```python
from build123d import *

# Parameters (mm, degrees)
F0_R     = 12
F0_R_2   = 10.25
F1_DEPTH = 270
F2_R     = 12
F3_DEPTH = 5
F4_R     = 12
F5_DEPTH = 5


with BuildPart() as f1:
    # F0 (on Front) → F1 (new body)
    with BuildSketch(Plane.XZ):
        Circle(F0_R)
        Circle(F0_R_2, mode=Mode.SUBTRACT)
    extrude(amount=F1_DEPTH)

    # F2 (on face) → F3 (join)
    with BuildSketch(Plane(origin=(0, 0, 0), x_dir=(-1, 0, 0), z_dir=(0, 1, 0))):
        Circle(F2_R)
    extrude(amount=F3_DEPTH)

    # F4 (on face) → F5 (join)
    with BuildSketch(Plane.XZ.offset(270)):
        Circle(F4_R)
    extrude(amount=F5_DEPTH)


solid = f1.part
```
Work out the finished part from the listing and answer in its coordinate system (mm). Round coordinates to 2 decimals unless told otherwise and drop trailing zeros. Write each loop counter-clockwise with the first axis right and the second up, starting at its lowest first coordinate (ties: lowest second). Pieces come first, ordered by that corner, then holes. Notation, with made-up numbers: (37, -3.5) -> (63, -3.5) arc R8 ccw to (63, 9.5) -> close; hole circle Ø8 at (-32, -40). An arc over 180 degrees is marked (long way). Write each question's results on one line, items separated by ' | '.
1) Flat-ended cylindrical pins translate along their axes: pin 1 (10 mm diameter, centred on x = -6, y = -130.5, fed in from +Z); pin 2 (3 mm diameter, centred on y = -151.5, z = 4, fed in from +X); pin 3 (1.5 mm diameter, centred on y = -186.5, z = -9, fed in from +X); pin 4 (3 mm diameter, centred on x = 9.5, z = 9.5, fed in from +Y). Find the tip coordinate at first contact, or state that the pin passes through.
Findings:
pin 1: stops at z = 11.96 | pin 2: stops at x = 11.74 | pin 3: stops at x = 8.71 | pin 4: stops at y = 5
2) The part is cut by section A-A (z = 0). Write down the section's boundary in (x, y).
Findings:
outline: (-12, -275) -> (12, -275) -> (12, 5) -> (-12, 5) -> close; hole (-10.25, -270) -> (10.25, -270) -> (10.25, 0) -> (-10.25, 0) -> close
3) The part is cut by section B-B (x = 0). Write down the section's boundary in (y, z), and give its area (4 significant figures).
Findings:
outline: (-275, -12) -> (5, -12) -> (5, 12) -> (-275, 12) -> close; hole (-270, -10.25) -> (0, -10.25) -> (0, 10.25) -> (-270, 10.25) -> close | area: 1,185 mm²
4) For a pull along Y with two mould halves and no side action, classify faces 1 (the flat face through (0, -275, 0)), 2 (the flat face through (0, -270, 0)), 3 (the flat face through (0, 5, 0)) as +Y half, -Y half, draft (parallel to the pull), parting line (faces both ways), or undercut.
Findings:
face 1: -Y half | face 2: undercut | face 3: +Y half
5) Consider line 1 along Z through (x, y) = (0, -151); line 2 along Y through (x, z) = (6, 2.25); line 3 along X through (y, z) = (-26.5, 5.75). Determine where each line is inside the solid, lowest interval first. Write a range as [from, to].
Findings:
line 1: z = [-12, -10.25], [10.25, 12] | line 2: y = [-275, -270], [0, 5] | line 3: x = [-10.53, -8.49], [8.49, 10.53]
6) The part is cut by section C-C (y = -62). Write down the section's boundary in (x, z), and give its area (3 significant figures).
Findings:
outline: circle Ø24 at (0, 0); hole circle Ø20.5 at (0, 0) | area: 122 mm²
